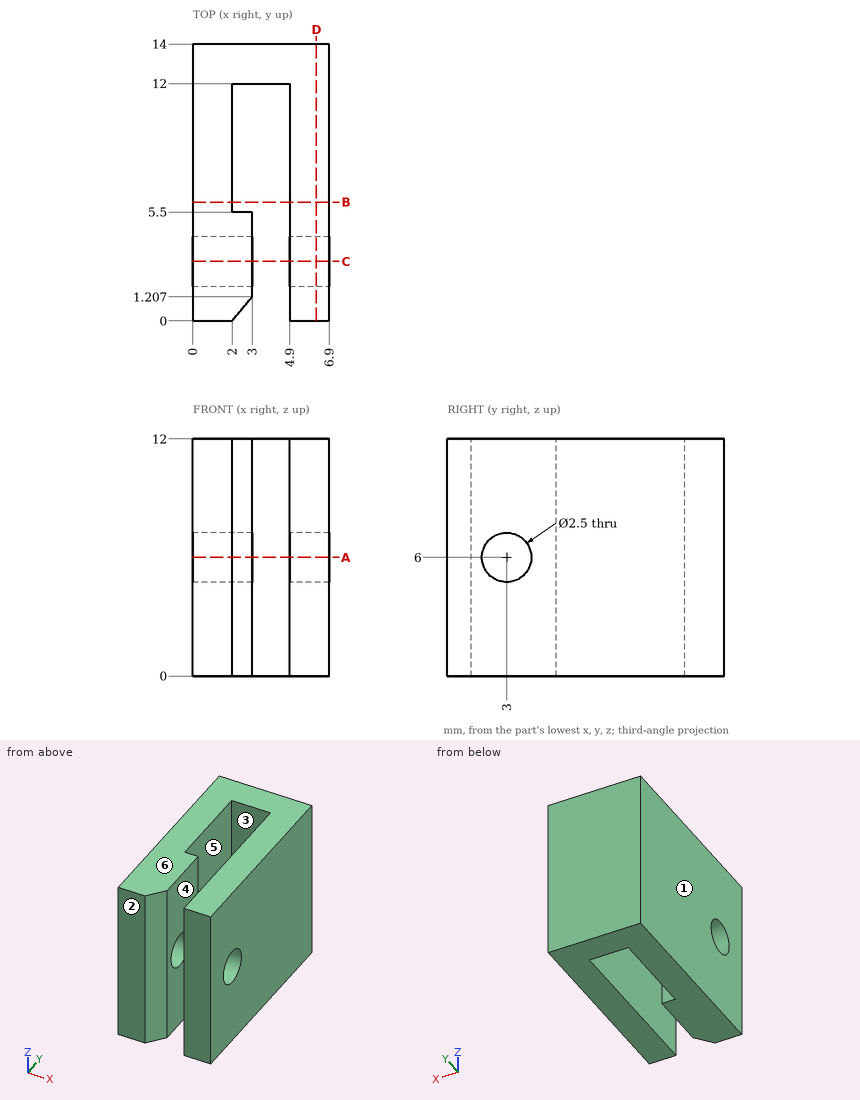
Design review of the part shown in the three views and the two pictorial views. Dimensions are in mm from the part's minimum x, y and z. A direction names the side the tool comes from. Round coordinates to 2 decimals unless told otherwise and drop trailing zeros. Order: outer loops, then holes, each group sorted by start corner. A loop starts at its lowest first (then second) coordinate and runs counter-clockwise, first axis right, second up.
Item 1: Draft analysis for pull direction X (two halves, no side actions). For the marked faces 1, 2 and 3, state which applies: released by +X, released by -X, zero draft, split by the parting line, or undercut.
Working result:
face 1: released by -X
face 2: zero draft
face 3: undercut
Item 2: Add section B-B, the plane y = 6. State the section outline as (x, z) points.
Working result:
outline: (0, 0) - (2, 0) - (2, 12) - (0, 12) - close; (4.9, 0) - (6.9, 0) - (6.9, 12) - (4.9, 12) - close
Item 3: For pin 1 (1.5 mm diameter, centred on y = 3, z = 6, fed in from -X), flat-tipped, find the tip position at first contact; note if it passes through.
Working result:
pin 1: passes through
Item 4: Machinability: for the marked faces 4, 5 and 6, which of the approach directions +Z, -Z, +X, -X, +Y, -Y give a long, thin tool a straight path to every point of the face, cutting with its end or side? Answer none if there is none.
Working result:
face 4: +Z, -Z, -Y
face 5: +Z, -Z
face 6: +Z, +X, -X, +Y, -Y
Item 5: To check wall thickness, follow probe 1 along X at (y, z) = (3.5, 8); probe 2 along Z at (x, y) = (2, 3); probe 3 along X at (y, z) = (11, 5). State the ranges of each line that lie inside material, in increasing order.
Working result:
probe 1: x = 0 to 3, 4.9 to 6.9
probe 2: z = 0 to 4.75, 7.25 to 12
probe 3: x = 0 to 2, 4.9 to 6.9
Item 6: Add section C-C, the plane y = 3. State the section outline as (x, z) points.
Working result:
outline: (0, 0) - (3, 0) - (3, 4.75) - (0, 4.75) - close; (0, 7.25) - (3, 7.25) - (3, 12) - (0, 12) - close; (4.9, 0) - (6.9, 0) - (6.9, 4.75) - (4.9, 4.75) - close; (4.9, 7.25) - (6.9, 7.25) - (6.9, 12) - (4.9, 12) - close
Item 7: Add section A-A, the plane z = 6. State the section outline as (x, y) points, and give its area (3 significant figures).
Working result:
outline: (0, 0) - (2, 0) - (3, 1.21) - (3, 1.75) - (0, 1.75) - close; (0, 4.25) - (3, 4.25) - (3, 5.5) - (2, 5.5) - (2, 12) - (4.9, 12) - (4.9, 4.25) - (6.9, 4.25) - (6.9, 14) - (0, 14) - close; (4.9, 0) - (6.9, 0) - (6.9, 1.75) - (4.9, 1.75) - close
area: 54.2 mm2
Item 8: Add section D-D, the plane x = 6.25. State the section outline as (y, z) points.
Working result:
outline: (0, 0) - (14, 0) - (14, 12) - (0, 12) - close; hole circle Ø2.5 at (3, 6)
